Could you check a few things on this model? Use its own coordinates, in mm. Give positions to 0.01 mm unless a question says otherwise; leave off trailing zeros. Loops run counter-clockwise (first coordinate to the right, second up) from the corner with the lowest first, then second, coordinate; pieces in that order, holes last. Notation, with made-up numbers: (79, 43.5) - (102, 43.5) arc R19 cw to (102, 65.5) - close; hole circle Ø6 at (3.25, -25). An arc over 180 degrees is marked (long way). Write each question's results on one line, items separated by ' | '. Start each with the question number.
(1) For pin 1 (1.5 mm diameter, centred on x = -22.5, y = 13.5, fed in from +Z); pin 2 (1 mm diameter, centred on x = -24, y = 12.5, fed in from -Z), each with a flat end and sliding along its axis, tell me the tip position at first contact or that it passes through.
(2) I need wall thicknesses on line 1 (Z direction, x = -24.65, y = 11.8); line 2 (Z direction, x = -23.75, y = 12.4); line 3 (X direction, y = 13.9, z = 5.25). Which ranges of each line are inside material? Lowest first, please.
(3) Suppose I cut it at A-A (y = 13.35). Please give me the cut outline in (x, z).
from build123d import *

# Parameters (mm, degrees)
SKETCH1_W          = 3
SKETCH1_H          = 3
EXTRUDE1_DEPTH     = 20
SKETCH2_OUTSIDE_W  = 9.09
SKETCH2_OUTSIDE_H  = 26.09
CUT_EXTRUDE1_DEPTH = 20
CHAMFER1_SIZE      = 0.2


with BuildPart() as part:
    # Sketch1 → Extrude1 (new body)
    with BuildSketch(Plane.XY):
        with Locations((-23.38908046, 12.550287356)):
            Rectangle(SKETCH1_W, SKETCH1_H)
    extrude(amount=EXTRUDE1_DEPTH)

    # Sketch2 outside → Cut-Extrude1 (cut)
    with BuildSketch(Plane(origin=(0, 14.050287356, 0), x_dir=(1, 0, 0), z_dir=(0, 1, 0))):
        with Locations((-23.389, -10)):
            Rectangle(SKETCH2_OUTSIDE_W, SKETCH2_OUTSIDE_H)
        with BuildLine():
            Line((-24.88908046, -1.5), (-24.88908046, -18.5))
            ThreePointArc((-24.88908046, -18.5), (-23.38908046, -20), (-21.88908046, -18.5))
            Line((-21.88908046, -18.5), (-21.88908046, -1.5))
            ThreePointArc((-21.88908046, -1.5), (-23.38908046, 0), (-24.88908046, -1.5))
        make_face(mode=Mode.SUBTRACT)
    extrude(amount=-CUT_EXTRUDE1_DEPTH, mode=Mode.SUBTRACT)

    # Chamfer1
    chamfer1_edges = [part.edges().sort_by_distance(p)[0] for p in [
        (-21.88908046, 14.050287356, 10),
        (-21.88908046, 11.050287356, 10),
        (-24.88908046, 11.050287356, 10),
        (-24.88908046, 14.050287356, 10),
        (-23.38908046, 14.050287356, 20),
        (-23.38908046, 14.050287356, 0),
        (-23.38908046, 11.050287356, 0),
        (-23.38908046, 11.050287356, 20),
    ]]
    chamfer(chamfer1_edges, length=CHAMFER1_SIZE)


solid = part.part
Output values:
1) pin 1: z = 19.99 | pin 2: z = 0
2) line 1: 0.69 to 19.31 | line 2: 0.04 to 19.96 | line 3: -24.84 to -21.94
3) outline: (-24.89, 1.5) arc R1.5 ccw to (-21.89, 1.5) - (-21.89, 18.5) arc R1.5 ccw to (-24.89, 18.5) - close
